Build history of the part. All positions in model axes, mm. A direction names the side the tool comes from. Round coordinates to 2 decimals unless told otherwise and drop trailing zeros. Write each loop counter-clockwise with the first axis right and the second up, starting at its lowest first coordinate (ties: lowest second). Pieces come first, ordered by that corner, then holes. Notation, with made-up numbers: (61.25, 49.25) -> (118.25, 49.25) arc R13 cw to (118.25, 72.25) -> close; hole circle Ø3 at (68, 26). An arc over 180 degrees is marked (long way). Answer in a Markdown table with one row per item.
```python
from build123d import *

# Parameters (mm, degrees)
SKETCH_1_W             = 89.5
SKETCH_1_H             = 69.5
EXTRUDE_1_DEPTH        = 99.5
SKETCH_2_W             = 10
SKETCH_2_H             = 15
CUT_EXTRUDE_1_DEPTH    = 1
FILLET_1_R             = 1
SKETCH_3_W             = 6.5
SKETCH_3_H             = 0.5
EXTRUDE_2_DEPTH        = 5
SKETCH_4_W             = 1
SKETCH_4_H             = 2
EXTRUDE_3_DEPTH        = 0.5
FILLET_2_R             = 1
FILLET_3_R             = 0.3
FILLET_2_OF_MIRROR_1_R = 1
FILLET_3_OF_MIRROR_1_R = 0.3
SKETCH_5_W             = 3.710206691
SKETCH_5_H             = 0.372043469
EXTRUDE_4_DEPTH        = 0.2
SKETCH_6_R             = 3.5
SKETCH_6_R_2           = 3.3
EXTRUDE_5_DEPTH        = 0.2


with BuildPart() as part:
    # 草图1 → 凸台-拉伸1 (new body)
    with BuildSketch(Plane(origin=(0, 0, 0), x_dir=(1, 0, 0), z_dir=(0, 1, 0))):
        Rectangle(SKETCH_1_W, SKETCH_1_H)
    extrude(amount=EXTRUDE_1_DEPTH)

    # 草图2 → 切除-拉伸1 (cut)
    with BuildSketch(Plane(origin=(0, 99.5, 0), x_dir=(1, 0, 0), z_dir=(0, 1, 0))):
        with Locations((-36.75, 25.25)):
            Rectangle(SKETCH_2_W, SKETCH_2_H)
        with Locations((36.75, 25.25)):
            Rectangle(SKETCH_2_W, SKETCH_2_H)
    extrude(amount=-CUT_EXTRUDE_1_DEPTH, mode=Mode.SUBTRACT)

    # 圆角1
    fillet_1_edges = [part.edges().sort_by_distance(p)[0] for p in [
        (-44.75, 99.5, 0),
        (0, 99.5, 34.75),
        (44.75, 99.5, 0),
        (0, 0, 34.75),
        (-44.75, 0, 0),
        (0, 0, -34.75),
        (44.75, 0, 0),
        (0, 99.5, -34.75),
        (44.75, 49.75, 34.75),
        (-44.75, 49.75, 34.75),
        (-44.75, 49.75, -34.75),
        (44.75, 49.75, -34.75),
    ]]
    fillet(fillet_1_edges, radius=FILLET_1_R)

    # 草图3 → 凸台-拉伸2 (add)
    with BuildSketch(Plane(origin=(0, 98.5, 0), x_dir=(1, 0, 0), z_dir=(0, 1, 0))):
        with Locations((36.75, 22)):
            Rectangle(SKETCH_3_W, SKETCH_3_H)
    extrude_2 = extrude(amount=EXTRUDE_2_DEPTH)

    # 草图4 → 凸台-拉伸3 (add)
    with BuildSketch(Plane(origin=(0, 103.5, 0), x_dir=(1, 0, 0), z_dir=(0, 1, 0))):
        Polygon((33.5, 21.75), (33.5, 19.25), (34.25, 19.25), (34.25, 14.25), (39.25, 14.25), (39.25, 19.25), (40, 19.25), (40, 21.75), align=None)
        with Locations((36.75, 16.75)):
            Rectangle(SKETCH_4_W, SKETCH_4_H, mode=Mode.SUBTRACT)
    extrude_3 = extrude(amount=-EXTRUDE_3_DEPTH)

    # 圆角2
    fillet_2_edges = [part.edges().sort_by_distance(p)[0] for p in [
        (36.75, 103.5, -22.25),
        (36.75, 103, -21.75),
    ]]
    fillet(fillet_2_edges, radius=FILLET_2_R)

    # 圆角3
    fillet_3_edges = [part.edges().sort_by_distance(p)[0] for p in [
        (40, 103.25, -19.25),
        (39.25, 103.25, -14.25),
        (34.25, 103.25, -14.25),
        (33.5, 103.25, -19.25),
    ]]
    fillet(fillet_3_edges, radius=FILLET_3_R)

    # 镜向1: 凸台-拉伸2, 凸台-拉伸3 across plane
    add(extrude_2.mirror(Plane(origin=(0, 0, 0), x_dir=(0, 0, 1), z_dir=(1, 0, 0))))
    add(extrude_3.mirror(Plane(origin=(0, 0, 0), x_dir=(0, 0, 1), z_dir=(1, 0, 0))))

    # 圆角2 of 镜向1
    fillet_2_of_mirror_1_edges = [part.edges().sort_by_distance(p)[0] for p in [
        (-36.75, 103.5, -22.25),
        (-36.75, 103, -21.75),
    ]]
    fillet(fillet_2_of_mirror_1_edges, radius=FILLET_2_OF_MIRROR_1_R)

    # 圆角3 of 镜向1
    fillet_3_of_mirror_1_edges = [part.edges().sort_by_distance(p)[0] for p in [
        (-40, 103.25, -19.25),
        (-39.25, 103.25, -14.25),
        (-34.25, 103.25, -14.25),
        (-33.5, 103.25, -19.25),
    ]]
    fillet(fillet_3_of_mirror_1_edges, radius=FILLET_3_OF_MIRROR_1_R)

    # 草图5 → 凸台-拉伸4 (add)
    with BuildSketch(Plane(origin=(0, 99.5, 0), x_dir=(1, 0, 0), z_dir=(0, 1, 0))):
        Polygon((21.528027711, 25.963655783), (21.528027711, 28.423489578), (21.78628469, 28.423489578), (21.78628469, 25.963655783), (23.512259546, 25.963655783), (23.512259546, 25.592890813), (21.78628469, 25.592890813), (21.78628469, 23.133057018), (21.528027711, 23.133057018), (21.528027711, 25.592890813), (19.802052855, 25.592890813), (19.802052855, 25.963655783), align=None)
        with Locations((-21.959689363, 25.792257863)):
            Rectangle(SKETCH_5_W, SKETCH_5_H)
    extrude(amount=EXTRUDE_4_DEPTH)

    # 草图6 → 凸台-拉伸5 (add)
    # profile 1 of 2: a face of its own
    with BuildSketch(Plane(origin=(0, 99.5, 0), x_dir=(1, 0, 0), z_dir=(0, 1, 0))):
        with Locations(Location((21.75, 25.75, 0), (0, 0, 90))):
            Circle(SKETCH_6_R)
        with Locations(Location((21.75, 25.75, 0), (0, 0, 270))):
            Circle(SKETCH_6_R_2, mode=Mode.SUBTRACT)
    # profile 2 of 2: a face of its own
    with BuildSketch(Plane(origin=(0, 99.5, 0), x_dir=(1, 0, 0), z_dir=(0, 1, 0))):
        with Locations(Location((-21.75, 25.75, 0), (0, 0, 90))):
            Circle(SKETCH_6_R)
        with Locations(Location((-21.75, 25.75, 0), (0, 0, 90))):
            Circle(SKETCH_6_R_2, mode=Mode.SUBTRACT)
    extrude(amount=EXTRUDE_5_DEPTH)


solid = part.part
```
Q1. Drop flat-ended pins along their axis: P1, Ø1.8, axis at x = -38.5, y = 100.5, coming from the +Z side; P2, Ø0.6, axis at x = 37.5, y = 103, coming from the +Z side; P3, Ø20, axis at x = 3, z = 4, coming from the +Y side. Give the stop position or say it passes through.
A:
| item | result |
|---|---|
| P1 | z = -21.75 |
| P2 | z = -14.25 |
| P3 | y = 99.5 |
Q2. Two-plate mould, pull along X, no slides. Class faces 1 (the flat face through (-1, 49, 34.75)), 2 (the flat face through (37, 100, -21.75)): released by +X, released by -X, zero draft, split by the parting line, or undercut.
A:
| item | result |
|---|---|
| face 1 | zero draft |
| face 2 | undercut |
Q3. Wall check: line 1 (X direction, y = 99.6, z = -25.75); line 2 (Z direction, x = -21.75, y = 99.55); line 3 (Y direction, x = -35.5, z = -14.5). Give the ranges that are in metal, low to high. Write a range as [from, to].
A:
| item | result |
|---|---|
| line 1 | [-25.25, -25.05], [-23.81, -20.1], [-18.45, -18.25], [18.25, 18.45], [19.8, 23.51], [25.05, 25.25] |
| line 2 | [-29.25, -29.05], [-25.98, -25.61], [-22.45, -22.25] |
| line 3 | [0, 99.5], [103, 103.5] |
Q4. Saw through at B-B on x = -28. Write the cut outline in (y, z).
A:
| item | result |
|---|---|
| outline | (0, -33.75) arc R1 ccw to (1, -34.75) -> (98.5, -34.75) arc R1 ccw to (99.5, -33.75) -> (99.5, 33.75) arc R1 ccw to (98.5, 34.75) -> (1, 34.75) arc R1 ccw to (0, 33.75) -> close |
Q5. Which spindle directions (+Z, -Z, +X, -X, +Y, -Y) get a long thin tool onto all of the face, cutting with end or side? Do faces 3 (the flat face through (37, 98.5, -25)), 4 (the flat face through (37, 103.5, -18)), 5 (the flat face through (-37, 103, -18)), 6 (the flat face through (40, 102, -22)), 7 (the flat face through (-1, 0, 0)). Say none if no direction does.
A:
| item | result |
|---|---|
| face 3 | none |
| face 4 | +Z, -Z, +X, -X, +Y |
| face 5 | +Z, +X, -X |
| face 6 | +Y |
| face 7 | +Z, -Z, +X, -X, -Y |
Q6. Saw through at A-A on z = -8.5. Write the cut outline in (x, y).
A:
| item | result |
|---|---|
| outline | (-44.75, 1) arc R1 ccw to (-43.75, 0) -> (43.75, 0) arc R1 ccw to (44.75, 1) -> (44.75, 98.5) arc R1 ccw to (43.75, 99.5) -> (-43.75, 99.5) arc R1 ccw to (-44.75, 98.5) -> close |
